Read the model definition and answer for the solid it produces. Units are mm, in the model's axes. A direction names the side the tool comes from. Coordinates: 2 decimals unless noted, no trailing zeros. Write each loop counter-clockwise with the first axis right and the second up, starting at its lowest first coordinate (ties: lowest second). Pieces come first, ordered by that corner, then holes. Notation, with made-up numbers: (64, 9.25) -> (119, 9.25) arc R14 cw to (119, 36.25) -> close; hole circle Ø5 at (-6, 76). An arc over 180 degrees is marked (long way). One line per item, written item: value. Start each with the question number.
1. Find section A-A, the plane x = -26.5. Write down the section's boundary in (y, z).
2. For faces 1 (the flat face through (-46, 90, 1)), 2 (the flat face through (-22, 60, 2)), determine the directions among +Z, -Z, +X, -X, +Y, -Y from which every point of the face is accessible in a straight line to the end or side of a thin tool.
3. Find section B-B, the plane y = 21. Write down the section's boundary in (x, z).
4. Consider line 1 along X through (y, z) = (53.5, 1.2); line 2 along Y through (x, z) = (-41.5, 2.6); line 3 along X through (y, z) = (18, 2.5). Determine where each line is inside the solid, lowest interval first.
5. Given P1, Ø1.5, axis at y = 38.5, z = 1.5, coming from the +X side, flat-ended and moving along its own axis, determine where the tip first touches the part or whether it passes through.
6. Find section D-D, the plane z = 0.5. Write down the section's boundary in (x, y).
7. Find section C-C, the plane y = 37.5. Write down the section's boundary in (x, z), and give its area (3 significant figures).
```python
from build123d import *

# Parameters (mm, degrees)
SKETCH_W     = 90
SKETCH_H     = 90
PAD_DEPTH    = 3
POCKET_DEPTH = 3


with BuildPart() as part:
    # Sketch → Pad (new body)
    with BuildSketch(Plane.XY):
        with Locations((-45, 45)):
            Rectangle(SKETCH_W, SKETCH_H)
    extrude(amount=PAD_DEPTH)

    # Sketch001 (on Face6 of Pad) → Pocket (cut)
    with BuildSketch(Plane.XY.offset(3)):
        Polygon((-75, 75), (-75, 15), (-15, 15), (-15, 60), (-30, 60), (-30, 30), (-60, 30), (-60, 75), align=None)
    extrude(amount=-POCKET_DEPTH, mode=Mode.SUBTRACT)


solid = part.part
```
Answer block:
1. outline: (0, 0) -> (15, 0) -> (15, 3) -> (0, 3) -> close; (60, 0) -> (90, 0) -> (90, 3) -> (60, 3) -> close
2. face 1: +Z, -Z, +X, -X, +Y
2. face 2: +Z, -Z
3. outline: (-90, 0) -> (-75, 0) -> (-75, 3) -> (-90, 3) -> close; (-15, 0) -> (0, 0) -> (0, 3) -> (-15, 3) -> close
4. line 1: x = -90 to -75, -60 to -30, -15 to 0
4. line 2: y = 0 to 15, 30 to 90
4. line 3: x = -90 to -75, -15 to 0
5. P1: stops at x = 0
6. outline: (-90, 0) -> (0, 0) -> (0, 90) -> (-90, 90) -> close; hole (-75, 15) -> (-15, 15) -> (-15, 60) -> (-30, 60) -> (-30, 30) -> (-60, 30) -> (-60, 75) -> (-75, 75) -> close
7. outline: (-90, 0) -> (-75, 0) -> (-75, 3) -> (-90, 3) -> close; (-60, 0) -> (-30, 0) -> (-30, 3) -> (-60, 3) -> close; (-15, 0) -> (0, 0) -> (0, 3) -> (-15, 3) -> close
7. area: 180 mm2
